Geometry check sheet. Reference: the model listing, model coordinates, mm. Face numbers are marked on the shaded views. Round coordinates to 2 decimals unless told otherwise and drop trailing zeros. Loops run counter-clockwise (first coordinate to the right, second up) from the corner with the lowest first, then second, coordinate; pieces in that order, holes last. Notation, with made-up numbers: (83.25, 27.5) -> (94.25, 27.5) arc R17 ccw to (94.25, 48.5) -> close; hole circle Ø5 at (74, -18). An arc over 180 degrees is marked (long way). Use one line per item in the form item = value.
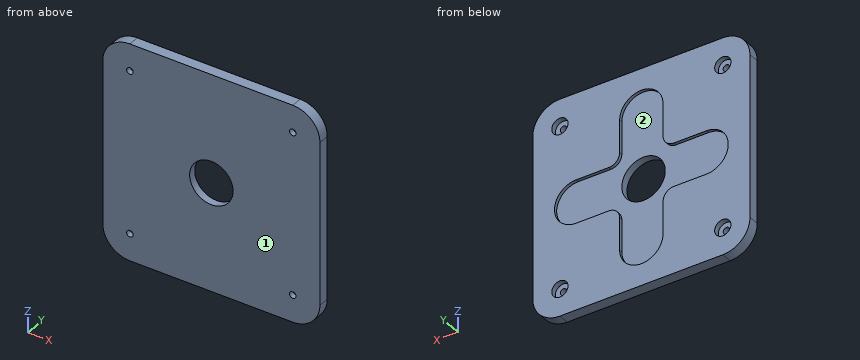
Autodesk Fusion 360 part; units mm, degrees
sketch "Boceto1" plane through (0, 0, 0) normal (0, 1, 0) x (1, 0, 0)
  line L0 (-75, 100) -> (75, 100)
  line L1 (100, 75) -> (100, -75)
  line L2 (75, -100) -> (-75, -100)
  line L3 (-100, -75) -> (-100, 75)
  line L4 (-100, 100) -> (100, -100) construction
  line L5 (100, 100) -> (-100, -100) construction
  arc A0 (-75, 100) -> (-100, 75) centre (-75, 75) ccw
  arc A1 (-100, -75) -> (-75, -100) centre (-75, -75) ccw
  arc A2 (75, -100) -> (100, -75) centre (75, -75) ccw
  arc A3 (100, 75) -> (75, 100) centre (75, 75) ccw
  circle A4 centre (-75, 75) radius 3
  circle A5 centre (75, 75) radius 3
  circle A6 centre (-75, -75) radius 3
  circle A7 centre (75, -75) radius 3
  circle A8 centre (-75, 75) radius 7.5
  circle A9 centre (75, 75) radius 7.5
  circle A10 centre (-75, -75) radius 7.5
  circle A11 centre (75, -75) radius 7.5
  line L6 (0, 0) -> (0, 60)
  line L7 (20, 0) -> (20, 60)
  line L8 (-20, 0) -> (-20, 60)
  line L9 (0, -20) -> (-60, -20)
  line L10 (0, 0) -> (-60, 0)
  line L11 (0, 20) -> (-60, 20)
  line L12 (20, 0) -> (20, -60)
  line L13 (0, 0) -> (0, -60)
  line L14 (-20, 0) -> (-20, -60)
  line L15 (0, 20) -> (60, 20)
  line L16 (0, 0) -> (60, 0)
  line L17 (0, -20) -> (60, -20)
  arc A12 (20, 60) -> (-20, 60) centre (0, 60) ccw
  arc A13 (-60, 20) -> (-60, -20) centre (-60, 0) ccw
  arc A14 (-20, -60) -> (20, -60) centre (0, -60) ccw
  arc A15 (60, -20) -> (60, 20) centre (60, 0) ccw
  circle A16 centre (0, 0) radius 20
  dimension "d1" = 200
  dimension "d2" = 200
  dimension "d3" = 25
  dimension "d4" = 6
  dimension "d5" = 6
  dimension "d6" = 6
  dimension "d7" = 6
  dimension "d8" = 15
  dimension "d9" = 15
  dimension "d10" = 15
  dimension "d11" = 15
  dimension "d12" = 60
  dimension "d13" = 20
  dimension "d14" = -20
  dimension "d16" = 360
  dimension "d18" = 360
  dimension "d25" = 40
extrude "Extruir1" add sketch "Boceto1" along normal blind 10 contours L0 L1 L2 L3 A0 A1 A2 A3
extrude "Extruir2" add sketch "Boceto1" along normal blind 7 contours L6 L10 A16 | L10 L13 A16 | L13 L16 A16 | L6 L16 A16 | L8 L11 A16 | L7 L8 L11 L15 A12 | L7 L15 A16 | L8 L9 L11 L14 A13 | L9 L14 A16 | L9 L12 L14 L17 A14 | L12 L17 A16 | L7 L12 L15 L17 A15
extrude "Extruir3" add sketch "Boceto1" along normal blind 5 contours A8 | A9 | A10 | A11
extrude "Extruir4" cut sketch "Boceto1" along normal blind 40 contours L6 L10 A16 | L10 L13 A16 | L13 L16 A16 | L6 L16 A16
fillet "Empalme1" radius 10 4 edges at (-20, 8.5, -20) (20, 8.5, -20) (-20, 8.5, 20) (20, 8.5, 20)
1. Gauge pin test, flat end, axial feed: pin 1 (9.5 mm diameter, centred on x = -75, z = 75, fed in from +Y). Record the tip position at first contact, or that the pin passes through.
Return value:
pin_1 = 5
2. Mould release check, pull along X, two halves, no side actions. Record for the marked faces 1 and 2: released by +X, released by -X, zero draft, split by the parting line, or undercut.
Return value:
face_1 = zero draft
face_2 = undercut
3. Material ranges on line 1 along Z through (x, y) = (-75, 3.75); line 2 along X through (y, z) = (6.25, -75); line 3 along X through (y, z) = (6.25, -0.5), recorded low to high.
Return value:
line_1 = -100 to -78, -72 to 72, 78 to 100
line_2 = -100 to -82.5, -67.5 to 67.5, 82.5 to 100
line_3 = -100 to -19.99, 19.99 to 100
4. Section check A-A (x = 16). Record the boundary of the cut face in (y, z).
Return value:
outline = (0, -100) -> (10, -100) -> (10, -72) -> (7, -72) -> (7, -12) -> (0, -12) -> close; (0, 12) -> (7, 12) -> (7, 72) -> (10, 72) -> (10, 100) -> (0, 100) -> close
5. Section check D-D (x = -50). Record the boundary of the cut face in (y, z), then the cut area to 3 significant figures.
Return value:
outline = (0, -100) -> (10, -100) -> (10, -20) -> (7, -20) -> (7, 20) -> (10, 20) -> (10, 100) -> (0, 100) -> close
area = 1,880 mm2
6. Section check C-C (z = -17.5). Record the boundary of the cut face in (x, y), then the cut area to 3 significant figures.
Return value:
outline = (-100, 0) -> (-9.68, 0) -> (-9.68, 7) -> (-69.68, 7) -> (-69.68, 10) -> (-100, 10) -> close; (9.68, 0) -> (100, 0) -> (100, 10) -> (69.68, 10) -> (69.68, 7) -> (9.68, 7) -> close
area = 1,450 mm2
7. Section check B-B (z = -57). Record the boundary of the cut face in (x, y).
Return value:
outline = (-100, 0) -> (100, 0) -> (100, 10) -> (20, 10) -> (20, 7) -> (-20, 7) -> (-20, 10) -> (-100, 10) -> close
